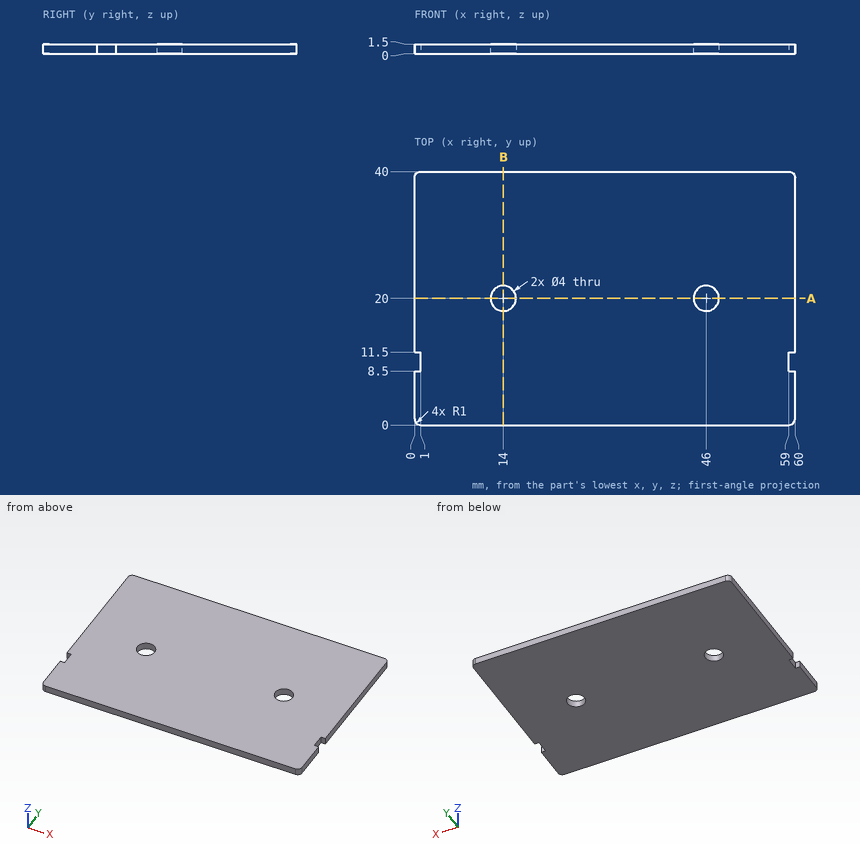
For this review, use the dimensioned drawing (mm, ordinates from the lowest corner) and the shaded views. Give positions to 0.01 mm unless a question says otherwise; leave off trailing zeros. Loops run counter-clockwise (first coordinate to the right, second up) from the corner with the lowest first, then second, coordinate; pieces in that order, holes last. Notation, with made-up numbers: (-25, -13.5) -> (2, -13.5) arc R18 cw to (2, 11.5) -> close; hole circle Ø3 at (28.5, -19.75). An arc over 180 degrees is marked (long way). Use CSV: the item, a comma, the result in double quotes.
1. Consider section B-B, the plane x = 14. Write out the cut boundary in (y, z).
Result:
outline,"(0, 0) -> (18, 0) -> (18, 1.5) -> (0, 1.5) -> close; (22, 0) -> (40, 0) -> (40, 1.5) -> (22, 1.5) -> close"
2. To check wall thickness, follow probe 1 along Y at (x, z) = (46, 0.3); probe 2 along Y at (x, z) = (47.5, 0.95). State the ranges of each line that lie inside material, in increasing order. Write a range as from..to.
Result:
probe 1,"y = 0..18, 22..40"
probe 2,"y = 0..18.68, 21.32..40"
3. Consider section A-A, the plane y = 20. Write out the cut boundary in (x, z).
Result:
outline,"(0, 0) -> (12, 0) -> (12, 1.5) -> (0, 1.5) -> close; (16, 0) -> (44, 0) -> (44, 1.5) -> (16, 1.5) -> close; (48, 0) -> (60, 0) -> (60, 1.5) -> (48, 1.5) -> close"
4. For P1, Ø0.5, axis at x = 0.5, z = 1, coming from the -Y side; P2, Ø0.5, axis at x = 59.5, z = 0.5, coming from the +Y side, all flat-tipped, find the tip position at first contact; note any pin that passes through.
Result:
P1,"stops at y = 0.03"
P2,"stops at y = 39.97"
